Source: CAD feature listing. Evaluate the final solid. Frame: model axes, mm. A direction names the side the tool comes from. Coordinates: 2 decimals unless noted, no trailing zeros. Order: outer loops, then holes, each group sorted by start corner. A loop starts at its lowest first (then second) coordinate and runs counter-clockwise, first axis right, second up.
Autodesk Inventor part; units mm, degrees
ref_plane "YZ Plane" through (0, 0, 0) normal (1, 0, 0) x (0, 1, 0)
ref_plane "XZ Plane" through (0, 0, 0) normal (0, 1, 0) x (-1, 0, 0)
ref_plane "XY Plane" through (0, 0, 0) normal (0, 0, 1) x (1, 0, 0)
sketch "Эскиз1" plane through (0, 0, 0) normal (0, 1, 0) x (-1, 0, 0)
  circle A0 centre (0, 0) radius 55
  dimension "d0" = 110
extrude "Выдавливание1" add sketch "Эскиз1" along normal mid plane 4
sketch "Эскиз2" plane through (0, 0, 0) normal (0, 1, 0) x (-1, 0, 0)
  circle A0 centre (0, 0) radius 55
  circle A1 centre (0, 0) radius 49.5
  circle A2 centre (0, 0) radius 45.5
  point P0 (0, 49.5)
  point P1 (0, 45.5)
  dimension "d4" = 99
  dimension "d5" = 4
extrude "Выдавливание2" add sketch "Эскиз2" along normal mid plane 12 contours A1
properties part number "внутреннее кольцо подшипника"
Q1. Set-up query: faces 4 (the flat face through (-22, 6, -40)), 5 (the cylindrical face through (6.44, 3.97, -49.08)), 6 (the cylindrical face through (6.44, -3.97, 49.08)). Return all of +Z, -Z, +X, -X, +Y, -Y with unobstructed straight access to the full face (end or side cutting, diameter ignored); none if empty.
Solutions:
face 4: +Z, -Z, +X, -X, +Y
face 5: +Y
face 6: -Y
Q2. Section query A-A on x = 0. Output: boundary loops of the cut face in (y, z).
Solutions:
outline: (-6, -49.5) - (-2, -49.5) - (-2, -55) - (2, -55) - (2, -49.5) - (6, -49.5) - (6, -45.5) - (2, -45.5) - (2, 45.5) - (6, 45.5) - (6, 49.5) - (2, 49.5) - (2, 55) - (-2, 55) - (-2, 49.5) - (-6, 49.5) - (-6, 45.5) - (-2, 45.5) - (-2, -45.5) - (-6, -45.5) - close
Q3. Pull-direction query (X, two-part tool) for faces 1 (the cylindrical face through (11.923, 0.028, -53.692)), 2 (the flat face through (45, 2, 21)), 3 (the cylindrical face through (36.107, -3.972, -27.686)); classes: pulls with the +X half, pulls with the -X half, needs draft (parallel to the pull), parting line crosses it, or undercut.
Solutions:
face 1: parting line crosses it
face 2: needs draft
face 3: undercut
Q4. Pin query (flat end, axial travel): P1, Ø3, axis at y = 4.5, z = -29.5, coming from the -X side; P2, Ø2, axis at x = -14.5, z = -10, coming from the -Y side; P3, Ø12, axis at x = 13, z = -27.5, coming from the +Y side. Return the tip coordinate at first contact, or that it passes through.
Solutions:
P1: stops at x = -40.82
P2: stops at y = -2
P3: stops at y = 2
Q5. Section query C-C on y = -4. Output: boundary loops of the cut face in (x, z).
Solutions:
outline: circle Ø99 at (0, 0); hole circle Ø91 at (0, 0)
Q6. Material intervals for line 1 along X through (y, z) = (4.75, 0); line 2 along Y through (x, z) = (20.5, 33), sorted ascending.
Solutions:
line 1: x = -49.5 to -45.5, 45.5 to 49.5
line 2: y = -2 to 2
Q7. Section query B-B on z = 0. Output: boundary loops of the cut face in (x, y), plus the area to 3 significant figures.
Solutions:
outline: (-55, -2) - (-49.5, -2) - (-49.5, -6) - (-45.5, -6) - (-45.5, -2) - (45.5, -2) - (45.5, -6) - (49.5, -6) - (49.5, -2) - (55, -2) - (55, 2) - (49.5, 2) - (49.5, 6) - (45.5, 6) - (45.5, 2) - (-45.5, 2) - (-45.5, 6) - (-49.5, 6) - (-49.5, 2) - (-55, 2) - close
area: 504 mm2
